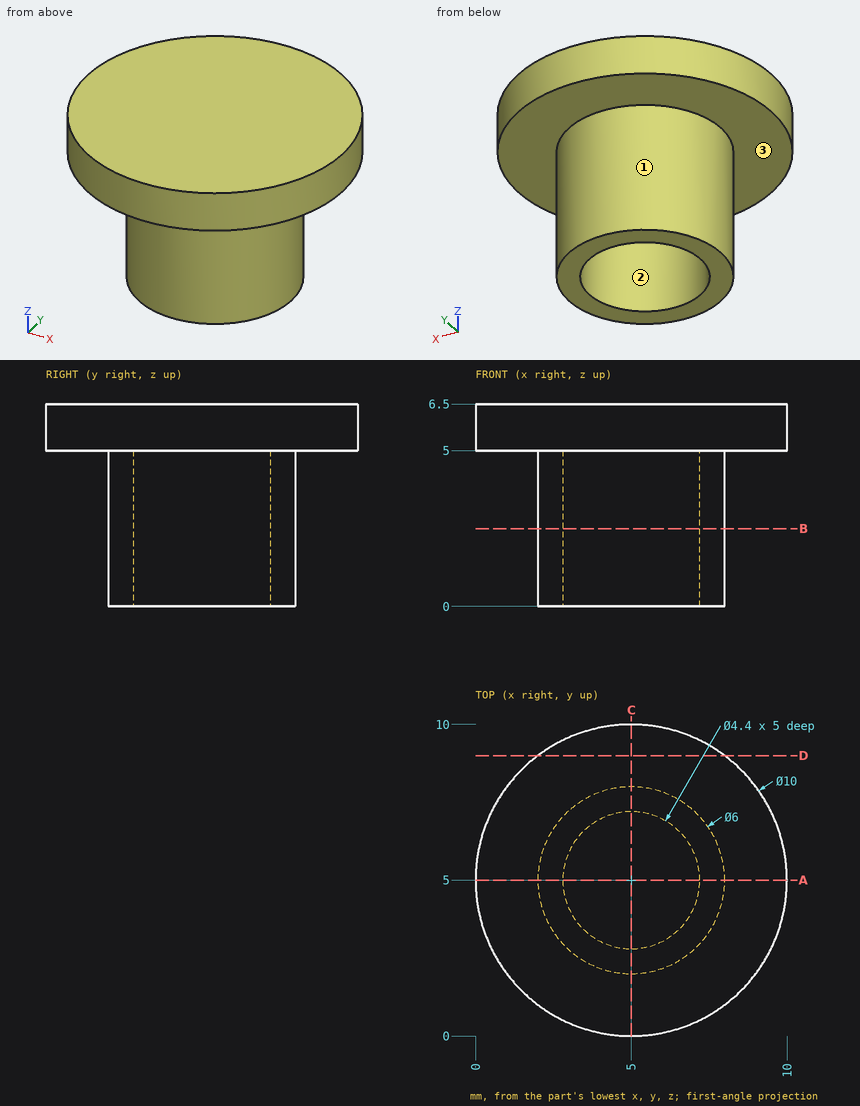
Print and shaded views of the part. All mm, measured from the part's lowest x, y and z. Coordinates: 2 decimals unless noted, no trailing zeros. Order: outer loops, then holes, each group sorted by start corner. A loop starts at its lowest first (then second) coordinate and runs counter-clockwise, first axis right, second up. Notation, with made-up numbers: (-10, -34) - (40, -34) arc R14 ccw to (40, -17) - close; hole circle Ø7 at (47, 25). An arc over 180 degrees is marked (long way). Put each result on its own line as item: value.
1. Saw through at D-D (y = 9). Write the cut outline in (x, z).
Answer sheet:
outline: (2, 5) - (8, 5) - (8, 6.5) - (2, 6.5) - close
2. Drop flat-ended pins along their axis: P1, Ø1.5, axis at x = 8, z = 5, coming from the +Y side; P2, Ø2, axis at x = 4, y = 5.5, coming from the -Z side. Give the stop position or say it passes through.
Answer sheet:
P1: stops at y = 9.47
P2: stops at z = 5
3. Pull direction X, two halves, no side cores. Call the marked faces 1, 2 and 3: pulls with the +X half, pulls with the -X half, needs draft (parallel to the pull), parting line crosses it, or undercut.
Answer sheet:
face 1: parting line crosses it
face 2: undercut
face 3: needs draft
4. Saw through at B-B (z = 2.5). Write the cut outline in (x, y), and give its area (3 significant figures).
Answer sheet:
outline: circle Ø6 at (5, 5); hole circle Ø4.4 at (5, 5)
area: 13.1 mm^2
5. Probe line 1 along Y through (x, z) = (5, 1.3); line 2 along Z through (x, y) = (2.5, 8.5); line 3 along Y through (x, z) = (4, 3.25). List the from-to ranges inside material, lowest first. Write a range as [from, to].
Answer sheet:
line 1: y = [2, 2.8], [7.2, 8]
line 2: z = [5, 6.5]
line 3: y = [2.17, 3.04], [6.96, 7.83]
6. Saw through at A-A (y = 5). Write the cut outline in (x, z).
Answer sheet:
outline: (0, 5) - (2, 5) - (2, 0) - (2.8, 0) - (2.8, 5) - (7.2, 5) - (7.2, 0) - (8, 0) - (8, 5) - (10, 5) - (10, 6.5) - (0, 6.5) - close
